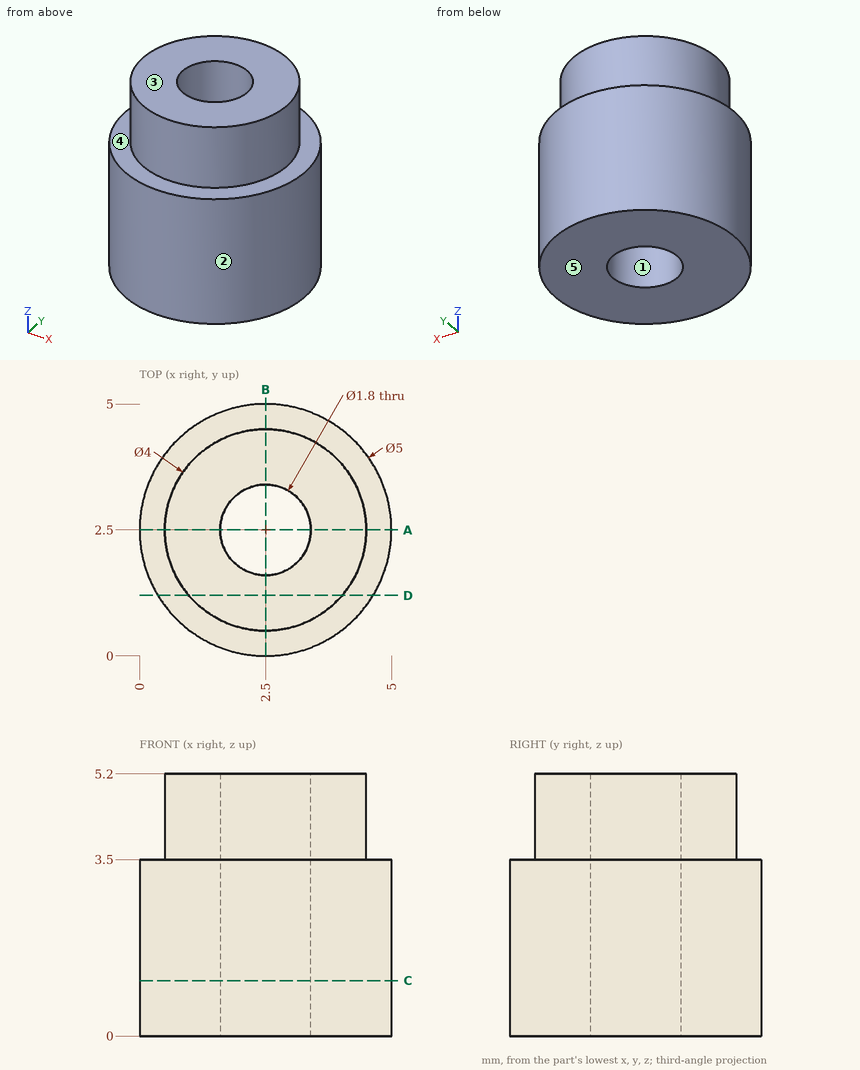
Study the drawing (mm; zero at the part's minimum x, y, z) and answer. A direction names the side the tool comes from. Coordinates: 2 decimals unless noted, no trailing zeros. Loops run counter-clockwise (first coordinate to the right, second up) from the corner with the lowest first, then second, coordinate; pieces in that order, holes last. Notation, with made-up numbers: M 29.25,53.25 L 37.25,53.25 A17 cw 37.25,81.25 Z; hole C 34.5,69.25 d1. An arc over 180 degrees is marked long. Answer as a JSON object with one key per item and string values. Group by question number.
Item 1: Section C-C (z = 1.1) is taken. Write down the section's boundary in (x, y), and give its area (3 significant figures).
Item 2: Consider L1, parallel to Y at x = 2.5, z = 2.8; L2, parallel to X at y = 3, z = 2.35; L3, parallel to Z at x = 2.7, y = 0.45. Determine where each line is inside the solid, lowest interval first.
Item 3: Section A-A (y = 2.5) is taken. Write down the section's boundary in (x, z), and give its area (3 significant figures).
Item 4: Which of the six approach directions +Z, -Z, +X, -X, +Y, -Y give full straight-line access (tool end or side, diameter ignored) to the marked faces 4 and 5?
Item 5: Each of these flat-tipped pins is pushed along its axis until it touches: P1, Ø2, axis at x = 4, z = 4, coming from the +Y side; P2, Ø1, axis at y = 4, z = 2.5, coming from the +X side. Where does it stop, or does it pass through?
Item 6: Determine the mould class of the marked faces 1, 2 and 3 for opening direction Y: +Y half, -Y half, draft (parallel to the pull), parting line (faces both ways), or undercut.
Item 7: Section D-D (y = 1.2) is taken. Write down the section's boundary in (x, z).
Solved:
{
 "1": {"outline": "C 2.5,2.5 d5; hole C 2.5,2.5 d1.8", "area": "17.1 mm2"},
 "2": {"L1": "y = 0 to 1.6, 3.4 to 5", "L2": "x = 0.05 to 1.75, 3.25 to 4.95", "L3": "z = 0 to 3.5"},
 "3": {"outline": "M 0,0 L 1.6,0 L 1.6,5.2 L 0.5,5.2 L 0.5,3.5 L 0,3.5 Z; M 3.4,0 L 5,0 L 5,3.5 L 4.5,3.5 L 4.5,5.2 L 3.4,5.2 Z", "area": "14.9 mm2"},
 "4": {"face 4": "+Z", "face 5": "-Z, +X, -X, +Y, -Y"},
 "5": {"P1": "stops at y = 4.92", "P2": "stops at x = 4.79"},
 "6": {"face 1": "undercut", "face 2": "parting line", "face 3": "draft"},
 "7": {"outline": "M 0.36,0 L 4.64,0 L 4.64,3.5 L 4.02,3.5 L 4.02,5.2 L 0.98,5.2 L 0.98,3.5 L 0.36,3.5 Z"}
}
